The model under review builds one solid part; all positions refer to its coordinate system, in mm. Face numbers are marked on the shaded views. Give positions to 0.01 mm unless a question says otherwise; leave off trailing zeros. Order: outer loops, then holes, each group sorted by start corner. A loop starts at its lowest first (then second) coordinate and runs counter-clockwise, first axis right, second up. Notation, with made-up numbers: (-29.5, 1) - (0.5, 1) arc R18 cw to (0.5, 35) - close; hole circle Ø9 at (37.5, 59). An arc over 180 degrees is marked (long way). Use CSV: the item, a comma, the result in double quotes. Start each with the question number.
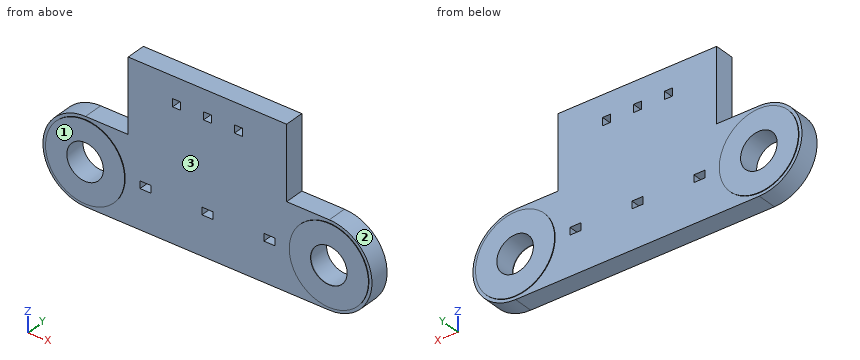
```python
from build123d import *
from build123d.topology import SkipClean

# Parameters (mm, degrees)
BOSS_EXTRUDE1_DEPTH      = 0.8
BOSS_EXTRUDE1_DEPTH_BACK = 0.8
SKETCH1_R                = 1.5
SKETCH4_R                = 3.25
SKETCH4_R_2              = 1.5
BOSS_EXTRUDE4_DEPTH      = 0.05
SKETCH5_W                = 0.64
SKETCH5_H                = 0.635
SKETCH5_H_2              = 0.64
CUT_EXTRUDE1_DEPTH       = 1.6
SKETCH6_W                = 0.9
SKETCH6_H                = 0.6
CUT_EXTRUDE2_DEPTH       = 1.6


with BuildPart() as part:
    # Sketch1 → Boss-Extrude1 (new, two sides: drawn at the far end of the back side and taken through both)
    with BuildSketch(Plane(origin=(0, 0, 0), x_dir=(1, 0, 0), z_dir=(0, 1, 0)).offset(-BOSS_EXTRUDE1_DEPTH_BACK)):
        with BuildLine():
            Line((-10, 3.5), (10, 3.5))
            ThreePointArc((10, 3.5), (13.5, 0), (10, -3.5))
            Line((10, -3.5), (6.5, -3.5))
            Line((6.5, -3.5), (6.5, -9.5))
            Line((6.5, -9.5), (-6.5, -9.5))
            Line((-6.5, -9.5), (-6.5, -3.5))
            Line((-6.5, -3.5), (-10, -3.5))
            ThreePointArc((-10, -3.5), (-13.5, 0), (-10, 3.5))
        make_face()
        with Locations(Location((-10, 0, 0), (0, 0, 270))):
            Circle(SKETCH1_R, mode=Mode.SUBTRACT)
        with Locations(Location((10, 0, 0), (0, 0, 90))):
            Circle(SKETCH1_R, mode=Mode.SUBTRACT)
    extrude(amount=BOSS_EXTRUDE1_DEPTH + BOSS_EXTRUDE1_DEPTH_BACK)

    # Sketch4 → Boss-Extrude4 (add)
    # profile 1 of 2: a face of its own
    with BuildSketch(Plane(origin=(0, 0.8, 0), x_dir=(1, 0, 0), z_dir=(0, 1, 0))):
        with Locations(Location((-10, 0, 0), (0, 0, 270))):
            Circle(SKETCH4_R)
        with Locations(Location((-10, 0, 0), (0, 0, 270))):
            Circle(SKETCH4_R_2, mode=Mode.SUBTRACT)
    # profile 2 of 2: a face of its own
    with BuildSketch(Plane(origin=(0, 0.8, 0), x_dir=(1, 0, 0), z_dir=(0, 1, 0))):
        with Locations(Location((10, 0, 0), (0, 0, 90))):
            Circle(SKETCH4_R)
        with Locations(Location((10, 0, 0), (0, 0, 270))):
            Circle(SKETCH4_R_2, mode=Mode.SUBTRACT)
    boss_extrude4 = extrude(amount=BOSS_EXTRUDE4_DEPTH)

    # Mirror1: Boss-Extrude4 across plane
    with SkipClean():  # the faces are left unmerged after this step: merging them gives an invalid solid
        add(boss_extrude4.mirror(Plane.ZX))

    # Sketch5 → Cut-Extrude1 (cut)
    with SkipClean():  # the faces are left unmerged after this step: merging them gives an invalid solid
        with BuildSketch(Plane(origin=(0, 0.8, 0), x_dir=(1, 0, 0), z_dir=(0, 1, 0))):
            with Locations((0, -7.4175)):
                Rectangle(SKETCH5_W, SKETCH5_H)
            with Locations((-2.54, -7.4175)):
                Rectangle(SKETCH5_W, SKETCH5_H_2)
            with Locations((2.54, -7.4175)):
                Rectangle(SKETCH5_W, SKETCH5_H_2)
        extrude(amount=-CUT_EXTRUDE1_DEPTH, mode=Mode.SUBTRACT)

    # Sketch6 → Cut-Extrude2 (cut)
    with SkipClean():  # the faces are left unmerged after this step: merging them gives an invalid solid
        with BuildSketch(Plane(origin=(0, 0.8, 0), x_dir=(1, 0, 0), z_dir=(0, 1, 0))):
            Rectangle(SKETCH6_W, SKETCH6_H)
            with Locations((-5.08, 0)):
                Rectangle(SKETCH6_W, SKETCH6_H)
            with Locations((5.08, 0)):
                Rectangle(SKETCH6_W, SKETCH6_H)
        extrude(amount=-CUT_EXTRUDE2_DEPTH, mode=Mode.SUBTRACT)


solid = part.part
```
1. Mouldability with a two-part tool opening along X and no side actions: class the marked faces 1, 2 and 3 as pulls with the +X half, pulls with the -X half, needs draft (parallel to the pull), parting line crosses it, or undercut.
2. Consider section B-B (z = 2). Give the boundary of the cut face in (x, y), and give its area (3 significant figures).
3. Consider section C-C (x = -8). Give the boundary of the cut face in (y, z).
4. Clearance check with flat-ended pins moving along their axes: pin 1 (4 mm diameter, centred on x = 1, z = 2, fed in from +Y); pin 2 (6.5 mm diameter, centred on x = -3.5, z = 5.5, fed in from -Y); pin 3 (0.5 mm diameter, centred on y = 0, z = 7.5, fed in from -X). State where each tip first meets the part, or that it passes through.
5. Consider section A-A (y = 0.5). State how many separate pieces and enclosed holes the cut face has, and give its area (3 significant figures).
6. To check wall thickness, follow L1, parallel to X at y = -0.75, z = 0; L2, parallel to Z at x = -0.25, y = -0.15 (3 decimals); L3, parallel to Z at x = 10, y = -0.5. State the ranges of each line that lie inside material, in increasing order. Write a range as [from, to].
Answers follow:
1,face 1,"needs draft"
1,face 2,"pulls with the +X half"
1,face 3,"undercut"
2,outline,"(-12.87, -0.8) - (-12.56, -0.8) - (-12.56, -0.85) - (-7.44, -0.85) - (-7.44, -0.8) - (7.44, -0.8) - (7.44, -0.85) - (12.56, -0.85) - (12.56, -0.8) - (12.87, -0.8) - (12.87, 0.8) - (12.56, 0.8) - (12.56, 0.85) - (7.44, 0.85) - (7.44, 0.8) - (-7.44, 0.8) - (-7.44, 0.85) - (-12.56, 0.85) - (-12.56, 0.8) - (-12.87, 0.8) - close"
2,area,"42.2 mm^2"
3,outline,"(-0.85, -2.56) - (-0.8, -2.56) - (-0.8, -3.5) - (0.8, -3.5) - (0.8, -2.56) - (0.85, -2.56) - (0.85, 2.56) - (0.8, 2.56) - (0.8, 3.5) - (-0.8, 3.5) - (-0.8, 2.56) - (-0.85, 2.56) - close"
4,pin 1,"stops at y = 0.8"
4,pin 2,"stops at y = -0.8"
4,pin 3,"stops at x = -6.5"
5,separate pieces,"1"
5,enclosed holes,"8"
5,area,"240 mm^2"
6,L1,"x = [-13.5, -11.5], [-8.5, -5.53], [-4.63, -0.45], [0.45, 4.63], [5.53, 8.5], [11.5, 13.5]"
6,L2,"z = [-3.5, -0.3], [0.3, 7.1], [7.735, 9.5]"
6,L3,"z = [-3.5, -1.5], [1.5, 3.5]"
